Work out the finished part from the listing and answer in its coordinate system (mm). A direction names the side the tool comes from. Give positions to 0.01 mm unless a question says otherwise; leave off trailing zeros. Order: outer loops, then holes, each group sorted by start corner. A loop starts at its lowest first (then second) coordinate and runs counter-clockwise, first axis right, second up. Notation, with made-up numbers: (62.5, 22.5) - (103.5, 22.5) arc R11 cw to (103.5, 26.5) - close; hole circle Ø6 at (31, -10). An arc over 180 degrees is marked (long way). Put each result on its own line as item: value.
Autodesk Inventor part; units mm, degrees
ref_plane "YZ Plane" through (0, 0, 0) normal (1, 0, 0) x (0, 1, 0)
ref_plane "XZ Plane" through (0, 0, 0) normal (0, 1, 0) x (-1, 0, 0)
ref_plane "XY Plane" through (0, 0, 0) normal (0, 0, 1) x (1, 0, 0)
sketch "Szkic1" plane through (0, 0, 0) normal (0, 0, 1) x (1, 0, 0)
  line L0 (0, 0) -> (0, 33.1)
  line L1 (0, 33.1) -> (5, 33.1)
  line L2 (5, 33.1) -> (5, -21)
  line L3 (-62.5, -3) -> (-62.5, 0)
  line L4 (-62.5, 0) -> (0, 0)
  line L5 (-62.5, -3) -> (-50.5, -3)
  line L6 (-50.5, -3) -> (-50.5, -18)
  line L7 (-50.5, -18) -> (-62.5, -18)
  line L8 (-62.5, -18) -> (-62.5, -21)
  line L9 (-62.5, -21) -> (5, -21)
  dimension "d1" = 15
  dimension "d3" = 3
  dimension "d4" = 12
  dimension "d6" = 3
  dimension "d7" = 5
  dimension "d8" = 33.1
  dimension "d9" = 50.5
extrude "Wyciągnięcie proste1" add sketch "Szkic1" along normal blind 25
sketch "Szkic2" plane through (-50.5, -18, 0) normal (-1, 0, 0) x (0, 0, 1)
  line L0 (0, 0) -> (0, 15) construction
  line L1 (0, 0) -> (25, 0) construction
  line L2 (25, 15) -> (25, 0) construction
  line L3 (0, 15) -> (25, 15) construction
  line L4 (0, 15) -> (12, 15)
  line L5 (12, 15) -> (12, 0)
  line L6 (12, 0) -> (0, 0)
  line L7 (0, 0) -> (0, 15)
  point P0 (0, 18)
  dimension "d14" = 13
extrude "Wyciągnięcie proste2" add sketch "Szkic2" along normal up to surface (12 mm away)
chamfer "Faza1" distance 9 angle 45 1 edges at (-62.5, -10.5, 0)
sketch "Szkic4" plane through (-62.5, -21, 25) normal (0, -1, 0) x (1, 0, 0)
  line L0 (0, 0) -> (67.5, 0) construction
  line L1 (62.5, 0) -> (0, 0) construction
  arc A0 (17.5, 0) -> (67.5, -14) centre (131.2021, 309.7932) ccw
  line L2 (67.5, 0) -> (67.5, -25) construction
  line L3 (62.5, -25) -> (67.5, -25) construction
  line L4 (17.5, 0) -> (67.5, 0)
  line L5 (67.5, 0) -> (67.5, -14)
  dimension "d21" = 11
  dimension "d23" = 50
  dimension "d24" = 330
extrude "Wyciągnięcie proste3" cut sketch "Szkic4" against normal up to surface (54.1 mm away)
fillet "Zaokrąglenie1" radius 1 8 edges at (5, -21, 5.5) (0, 0, 6.012) (5, 33.1, 5.5) (0, 33.1, 6.012) (-62.5, 0, 17) (-62.5, -21, 17) (-62.5, -18, 18.5) (-62.5, -3, 18.5)
equation "\"d3\" = d2"
properties part number "CH_01_0024_piston_adapter"
(1) A tool of negligible diameter and unlimited length cuts with its end or side. For faces 4 (the face through (-62.5, -11.2, 11.6)), 5 (the face through (-50.5, -10, 18)), 6 (the face through (0, 16, 6)), from which of +Z, -Z, +X, -X, +Y, -Y can it reach the whole face along a straight path? Write none if from no direction.
Geometry check:
face 4: +Z, -Z, -X, +Y, -Y
face 5: +Z, -X
face 6: +Z, -Z, -X, +Y
(2) Given pin 1 (12 mm diameter, centred on x = -30.5, z = 4.5, fed in from +Y); pin 2 (4 mm diameter, centred on y = 3, z = 12.5, fed in from +X); pin 3 (3.5 mm diameter, centred on x = -57, y = -8, fed in from +Z); pin 4 (6.5 mm diameter, centred on y = -13, z = 19, fed in from -X), each flat-ended and moving along its own axis, determine where each tip first touches the part or whether it passes through.
Geometry check:
pin 1: stops at y = 0
pin 2: stops at x = 5
pin 3: stops at z = 12
pin 4: stops at x = -50.5
(3) Section B-B, the plane x = -51.5 is taken. Write down the section's boundary in (y, z).
Geometry check:
outline: (-21, 0) - (0, 0) - (0, 25) - (-3, 25) - (-3, 12) - (-18, 12) - (-18, 25) - (-21, 25) - close
(4) Section D-D, the plane z = 19.5 is taken. Write down the section's boundary in (x, y), then the cut area to 3 significant figures.
Geometry check:
outline: (-62.5, -20) arc R1 ccw to (-61.5, -21) - (-28.72, -21) - (-28.72, 0) - (-61.5, 0) arc R1 ccw to (-62.5, -1) - (-62.5, -2) arc R1 ccw to (-61.5, -3) - (-50.5, -3) - (-50.5, -18) - (-61.5, -18) arc R1 ccw to (-62.5, -19) - close
area: 529 mm²
(5) Straight lines are drawn through the part: line 1 (Z direction, x = -53, y = -11.5); line 2 (Y direction, x = -51, z = 15); line 3 (Y direction, x = -12, z = 7.75). For each, find the intervals that lie inside material, in ascending order.
Geometry check:
line 1: z = 0 to 12
line 2: y = -21 to -18, -3 to 0
line 3: y = -21 to 0
(6) Section A-A, the plane z = 4.25 is taken. Write down the section's boundary in (x, y), then the cut area to 3 significant figures.
Geometry check:
outline: (-57.75, -21) - (4, -21) arc R1 ccw to (5, -20) - (5, 32.1) arc R1 ccw to (4, 33.1) - (1, 33.1) arc R1 ccw to (0, 32.1) - (0, 1) arc R1 cw to (-1, 0) - (-57.75, 0) - close
area: 1,480 mm²
(7) Determine the mould class of faces 1 (the face through (-56, -3, 18)), 2 (the face through (-32, 0, 10)), 3 (the face through (-18, -6, 0)) for opening direction Y: pulls with the +Y half, pulls with the -Y half, needs draft (parallel to the pull), parting line crosses it, or undercut.
Geometry check:
face 1: undercut
face 2: pulls with the +Y half
face 3: needs draft
(8) Section C-C, the plane y = -6.5 is taken. Write down the section's boundary in (x, z).
Geometry check:
outline: (-62.5, 9) - (-53.5, 0) - (5, 0) - (5, 11) arc R330 cw to (-45, 25) - (-50.5, 25) - (-50.5, 12) - (-62.5, 12) - close
